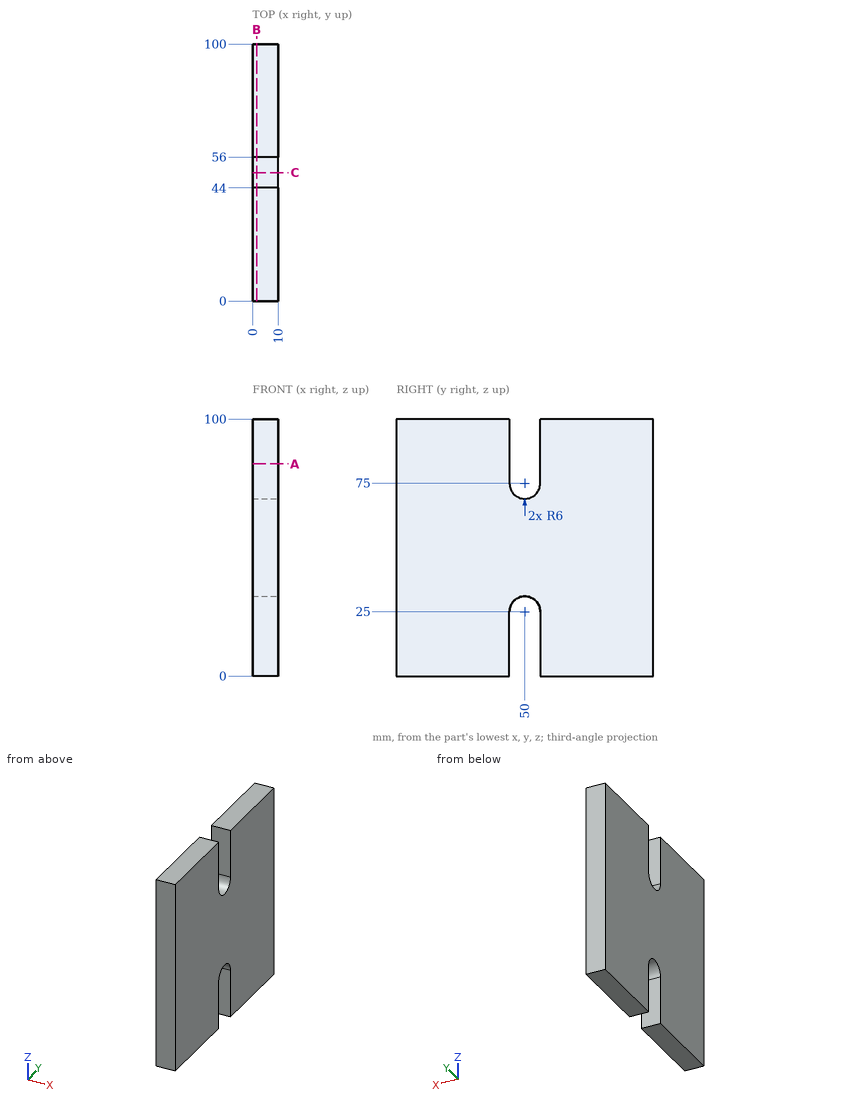
Geometry: see drawing. Coordinates: mm, zero at the bounding-box minimum. Coordinates: 2 decimals unless noted, no trailing zeros. Order: outer loops, then holes, each group sorted by start corner. A loop starts at its lowest first (then second) coordinate and runs counter-clockwise, first axis right, second up. Notation, with made-up numbers: (15, 75) - (43, 75) arc R26 ccw to (43, 95) - close; hole circle Ø6 at (-23.5, 48). An arc over 180 degrees is marked (long way). Use one line per item in the form item = value.
1) Section B-B (x = 1.5). Return loops of the section in (y, z), then the cut area to 3 significant figures.
Solutions:
outline = (0, 0) - (44, 0) - (44, 25) arc R6 cw to (56, 25) - (56, 0) - (100, 0) - (100, 100) - (56, 100) - (56, 75) arc R6 cw to (44, 75) - (44, 100) - (0, 100) - close
area = 9,290 mm^2
2) Section A-A (z = 82.5). Return loops of the section in (x, y), then the cut area to 3 significant figures.
Solutions:
outline = (0, 0) - (10, 0) - (10, 44) - (0, 44) - close; (0, 56) - (10, 56) - (10, 100) - (0, 100) - close
area = 880 mm^2
3) Section C-C (y = 50). Return loops of the section in (x, z), then the cut area to 3 significant figures.
Solutions:
outline = (0, 31) - (10, 31) - (10, 69) - (0, 69) - close
area = 380 mm^2
4) Ray query, L1, parallel to Y at x = 2.25, z = 86.5; L2, parallel to Z at x = 8.25, y = 49.5; L3, parallel to Y at x = 4.75, z = 30. Return the intervals inside material, ascending.
Solutions:
L1 = 0 to 44, 56 to 100
L2 = 30.98 to 69.02
L3 = 0 to 46.68, 53.32 to 100
